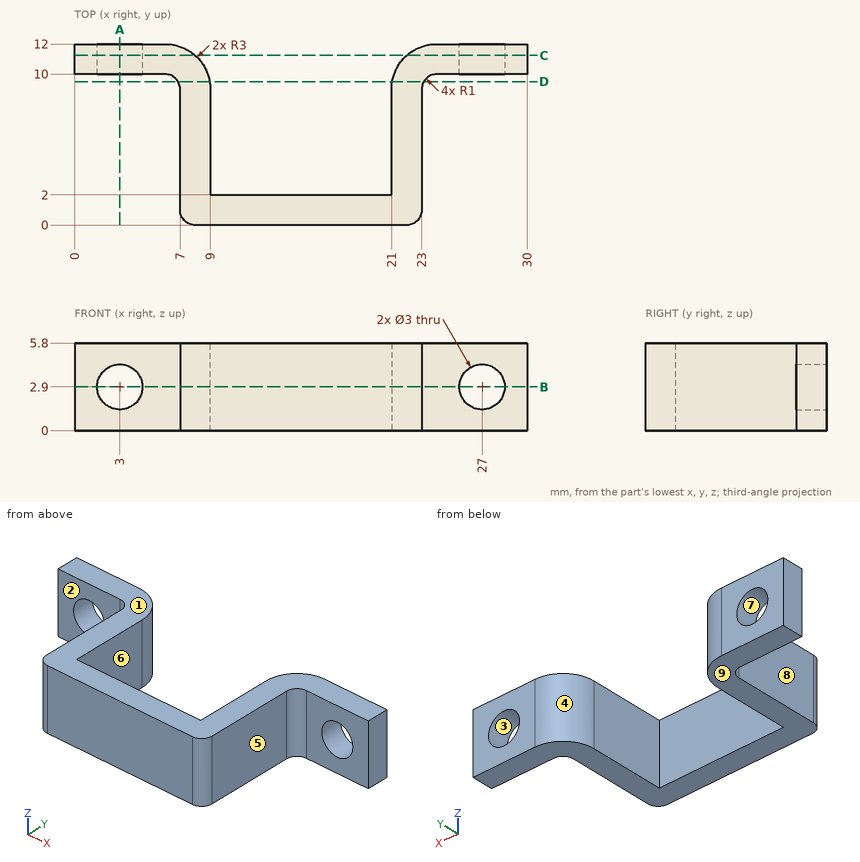
Answer from the drawing. Dimensions are ordinates in mm from the lowest x, y and z of the part. A direction names the side the tool comes from. Coordinates: 2 decimals unless noted, no trailing zeros. Loops run counter-clockwise (first coordinate to the right, second up) from the corner with the lowest first, then second, coordinate; pieces in that order, holes last.
1) Section D-D (y = 9.5) is taken. Give the vertices of the cut face in (x, z).
Results:
outline: (6.87, 0) - (8.96, 0) - (8.96, 5.8) - (6.87, 5.8) - close; (21.04, 0) - (23.13, 0) - (23.13, 5.8) - (21.04, 5.8) - close
2) Section C-C (y = 11.25) is taken. Give the vertices of the cut face in (x, z).
Results:
outline: (0, 0) - (7.98, 0) - (7.98, 5.8) - (0, 5.8) - close; (22.02, 0) - (30, 0) - (30, 5.8) - (22.02, 5.8) - close; hole circle Ø3 at (3, 2.9); hole circle Ø3 at (27, 2.9)
3) Section A-A (x = 3) is taken. Give the vertices of the cut face in (y, z), plus the area to 3 significant figures.
Results:
outline: (10, 0) - (12, 0) - (12, 1.4) - (10, 1.4) - close; (10, 4.4) - (12, 4.4) - (12, 5.8) - (10, 5.8) - close
area: 5.60 mm2
4) For the marked faces 1, 2, 3, 4 and 5, determine the directions among +Z, -Z, +X, -X, +Y, -Y from which every point of the face is accessible in a straight line to the end or side of a thin tool.
Results:
face 1: +Z, +X, -X, +Y, -Y
face 2: +Z, -Z, -X, -Y
face 3: +Y, -Y
face 4: +Z, -Z, +Y
face 5: +Z, -Z, +X, -Y
5) Flat-ended cylindrical pins translate along their axes: pin 1 (1.8 mm diameter, centred on x = 3, z = 2.9, fed in from -Y); pin 2 (3 mm diameter, centred on y = 2, z = 5, fed in from -X); pin 3 (3 mm diameter, centred on x = 16.5, z = 3, fed in from +Y); pin 4 (1.7 mm diameter, centred on y = 6, z = 2.5, fed in from +X). Find the tip coordinate at first contact, or state that the pin passes through.
Results:
pin 1: passes through
pin 2: stops at x = 7
pin 3: stops at y = 2
pin 4: stops at x = 23
6) Section B-B (z = 2.9) is taken. Give the vertices of the cut face in (x, y).
Results:
outline: (0, 10) - (1.5, 10) - (1.5, 12) - (0, 12) - close; (4.5, 10) - (6, 10) arc R1 cw to (7, 9) - (7, 1) arc R1 ccw to (8, 0) - (22, 0) arc R1 ccw to (23, 1) - (23, 9) arc R1 cw to (24, 10) - (25.5, 10) - (25.5, 12) - (24, 12) arc R3 ccw to (21, 9) - (21, 2) - (9, 2) - (9, 9) arc R3 ccw to (6, 12) - (4.5, 12) - close; (28.5, 10) - (30, 10) - (30, 12) - (28.5, 12) - close
7) For a pull along X with two mould halves and no side action, classify the marked faces 6, 7, 8 and 9 as +X half, -X half, draft (parallel to the pull), parting line (faces both ways), or undercut.
Results:
face 6: undercut
face 7: undercut
face 8: -X half
face 9: draft
8) Consider probe 1 along Z at (x, y) = (3, 10.8); probe 2 along X at (y, z) = (10.95, 2.9); probe 3 along X at (y, z) = (5.75, 3.05). Determine where each line is inside the solid, lowest interval first.
Results:
probe 1: z = 0 to 1.4, 4.4 to 5.8
probe 2: x = 0 to 1.5, 4.5 to 8.28, 21.72 to 25.5, 28.5 to 30
probe 3: x = 7 to 9, 21 to 23
